The model under review builds one solid part; all positions refer to its coordinate system, in mm. Round coordinates to 2 decimals unless told otherwise and drop trailing zeros. Write each loop counter-clockwise with the first axis right and the second up, starting at its lowest first coordinate (ties: lowest second). Pieces come first, ordered by that corner, then holes. Notation, with made-up numbers: M 12,70 L 55,70 A31 cw 55,105 Z; hole C 79.25,31.25 d9. An arc over 180 degrees is marked long. One line per item, written item: value. Start each with the question number.
1) Take a section at A-A, the plane x = -17. Write out the cut boundary in (y, z), and give its area (3 significant figures).
2) Take a section at B-B, the plane x = -33. Write out the cut boundary in (y, z).
3) For P1, Ø14, axis at x = -14.5, y = -31.5, coming from the -Z side; P2, Ø5.5, axis at y = -3, z = 130.5, coming from the +X side; P3, Ø2.5, axis at y = -3.5, z = -124.5, coming from the -X side, all flat-tipped, find the tip position at first contact; note any pin that passes through.
4) Wall thickness on probe 1 along Z at (x, y) = (-13.5, -11.5); probe 2 along Y at (x, z) = (-18, -122): over which ranges is each line inside the solid? List them lowest first.
from build123d import *

# Parameters (mm, degrees)
F1_DEPTH = 5
F2_DEPTH = 46


with BuildPart() as f1:
    # F0 (on Front) → F1 (new body)
    with BuildSketch(Plane.XZ):
        with BuildLine():
            Line((0, 119.5), (25, 119.5))
            Line((25, 119.5), (25, 133))
            Line((25, 133), (19.5, 133))
            Line((19.5, 133), (19.5, 127))
            ThreePointArc((19.5, 127), (17, 124.5), (14.5, 127))
            Line((14.5, 127), (14.5, 133))
            Line((14.5, 133), (0, 133))
            Line((0, 133), (-14.5, 133))
            Line((-14.5, 133), (-14.5, 127))
            ThreePointArc((-14.5, 127), (-17, 124.5), (-19.5, 127))
            Line((-19.5, 127), (-19.5, 133))
            Line((-19.5, 133), (-25, 133))
            Line((-25, 133), (-25, 119.5))
            Line((-25, 119.5), (0, 119.5))
        make_face()
    extrude(amount=F1_DEPTH)



with BuildPart() as f1b:
    # F0 (on Front) → F1, piece 2 (new body)
    with BuildSketch(Plane.XZ):
        with BuildLine():
            Line((25, -133), (25, -119.5))
            Line((25, -119.5), (0, -119.5))
            Line((0, -119.5), (-25, -119.5))
            Line((-25, -119.5), (-25, -133))
            Line((-25, -133), (-19.5, -133))
            Line((-19.5, -133), (-19.5, -127))
            ThreePointArc((-19.5, -127), (-17, -124.5), (-14.5, -127))
            Line((-14.5, -127), (-14.5, -133))
            Line((-14.5, -133), (0, -133))
            Line((0, -133), (14.5, -133))
            Line((14.5, -133), (14.5, -127))
            ThreePointArc((14.5, -127), (17, -124.5), (19.5, -127))
            Line((19.5, -127), (19.5, -133))
            Line((19.5, -133), (25, -133))
        make_face()
    extrude(amount=F1_DEPTH)


with BuildPart() as f1_1:
    add(f1.part)

    add(f1b.part)  # F2 merges F1b
    # F0 (on Front) → F2 (join)
    with BuildSketch(Plane.XZ):
        Polygon((39.75, -119.5), (39.75, 0), (39.75, 119.5), (25, 119.5), (0, 119.5), (-25, 119.5), (-39.75, 119.5), (-39.75, 0), (-39.75, -119.5), (-25, -119.5), (0, -119.5), (25, -119.5), align=None)
    extrude(amount=F2_DEPTH)


solid = f1_1.part
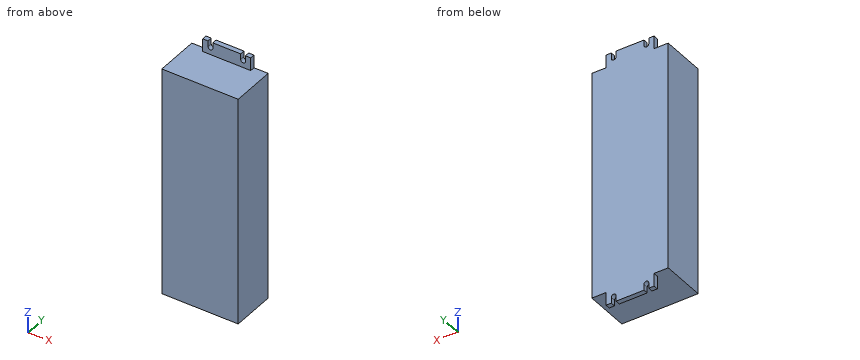
Checked values:
1. outline: M -46,-119.5 L -5,-119.5 L -5,-124.5 L 0,-124.5 L 0,124.5 L -5,124.5 L -5,119.5 L -46,119.5 Z
1. area: 11,000 mm2
2. outline: M -46,-119.5 L 0,-119.5 L 0,119.5 L -46,119.5 Z
3. P1: stops at z = -119.5
3. P2: stops at x = 25
3. P3: stops at x = -25
4. probe 1: z = -119.5 to 119.5
4. probe 2: y = -5 to 0
